```python
from build123d import *

# Parameters (mm, degrees)
CROQUIS1_W              = 3.5
CROQUIS1_H              = 3.5
SALIENTE_EXTRUIR1_DEPTH = 19
CROQUIS2_R              = 1
SALIENTE_EXTRUIR2_DEPTH = 2
SALIENTE_EXTRUIR3_START = 2
CROQUIS3_R              = 1
SALIENTE_EXTRUIR3_DEPTH = 2


with BuildPart() as part:
    # Croquis1 → Saliente-Extruir1 (new body)
    with BuildSketch(Plane.XY):
        Rectangle(CROQUIS1_W, CROQUIS1_H)
    extrude(amount=SALIENTE_EXTRUIR1_DEPTH)

    # Croquis2 → Saliente-Extruir2 (add)
    with BuildSketch(Plane.XY.offset(19)):
        with Locations(Location((0, 0, 0), (0, 0, 180))):
            Circle(CROQUIS2_R)
    extrude(amount=SALIENTE_EXTRUIR2_DEPTH)

    # Croquis3 → Saliente-Extruir3 (add)
    with BuildSketch(Plane(origin=(0, 0, 0), x_dir=(-1, 0, 0), z_dir=(0, 0, -1)).offset(SALIENTE_EXTRUIR3_START)):
        Circle(CROQUIS3_R)
    extrude(amount=-SALIENTE_EXTRUIR3_DEPTH)


solid = part.part
```
Design review of the part built by this model. Coordinates are the model's own, in mm. A direction names the side the tool comes from. Give positions to 0.01 mm unless a question says otherwise; leave off trailing zeros. Order: outer loops, then holes, each group sorted by start corner. A loop starts at its lowest first (then second) coordinate and runs counter-clockwise, first axis right, second up. Notation, with made-up numbers: (27, 51.5) -> (82, 51.5) arc R14 ccw to (82, 63.5) -> close; hole circle Ø2 at (63.5, 65). An arc over 180 degrees is marked (long way). Write item = value, one per line. Start each with the question number.
(1) We need section A-A on y = 0. Write out the cut boundary in (x, z).
(2) To check wall thickness, follow line 1 along Z through (x, y) = (0.8, 0.8); line 2 along Y through (x, z) = (-0.3, -0.5). State the ranges of each line that lie inside material, in increasing order.
(3) For faces 1 (the face through (0, 0, 21)), 2 (the face through (-1, -1, 0)), 3 (the face through (-1, -1, 19)), list the 3-axis set-ups (+Z, -Z, +X, -X, +Y, -Y) from which the entire face can be reached by the end or side of a thin tool; tool diameter is ignored.
Numbers:
q1.outline = (-1.75, 0) -> (-1, 0) -> (-1, -2) -> (1, -2) -> (1, 0) -> (1.75, 0) -> (1.75, 19) -> (1, 19) -> (1, 21) -> (-1, 21) -> (-1, 19) -> (-1.75, 19) -> close
q2.line_1 = 0 to 19
q2.line_2 = -0.95 to 0.95
q3.face_1 = +Z, +X, -X, +Y, -Y
q3.face_2 = -Z
q3.face_3 = +Z
